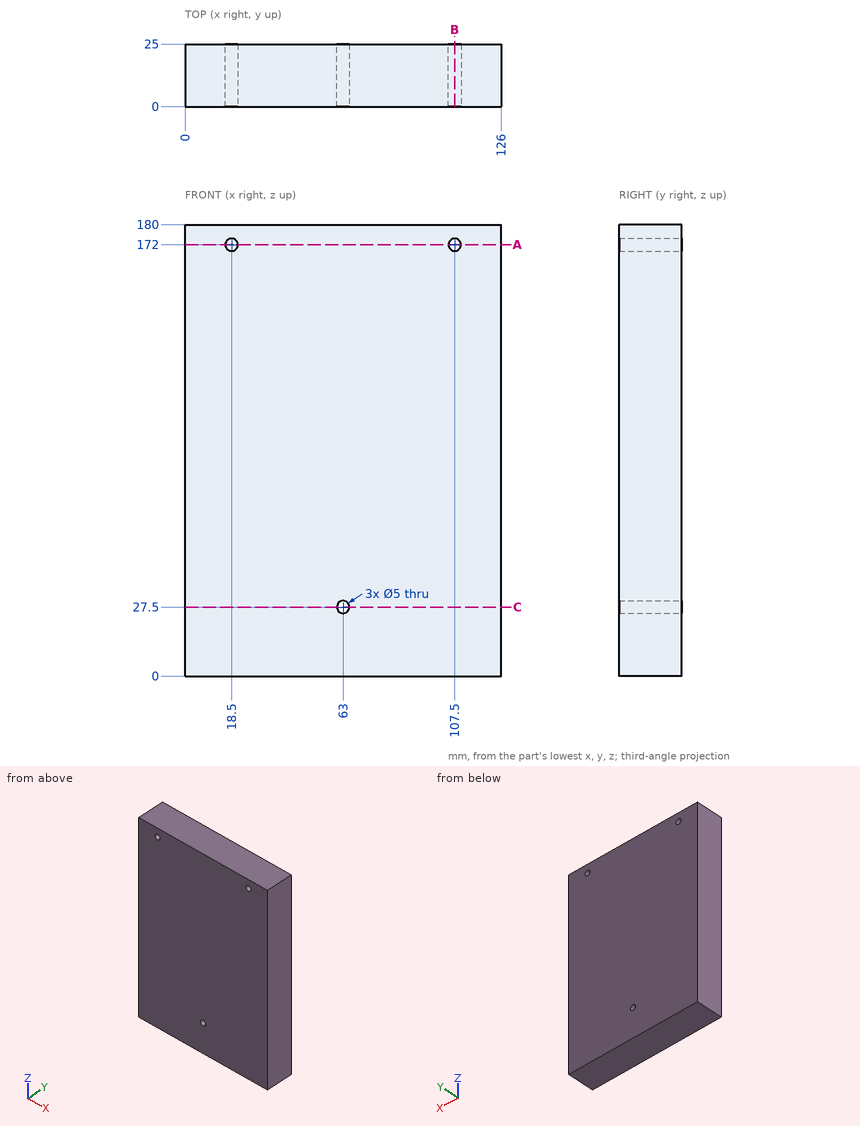
Part print with two shaded views. Sizes in mm from the minimum x, y, z corner. Give positions to 0.01 mm unless a question says otherwise; leave off trailing zeros. Loops run counter-clockwise (first coordinate to the right, second up) from the corner with the lowest first, then second, coordinate; pieces in that order, holes last. Notation, with made-up numbers: (-29.75, 69.5) -> (-9.75, 69.5) arc R33 ccw to (-9.75, 102.5) -> close; hole circle Ø9 at (-28.75, 2). An arc over 180 degrees is marked (long way). One line per question, with ' | ' between items.
Q1. Cut at C-C, the plane z = 27.5. Write the cut outline in (x, y).
Filled sheet:
outline: (0, 0) -> (60.5, 0) -> (60.5, 25) -> (0, 25) -> close; (65.5, 0) -> (126, 0) -> (126, 25) -> (65.5, 25) -> close
Q2. Cut at B-B, the plane x = 107.5. Write the cut outline in (y, z).
Filled sheet:
outline: (0, 0) -> (25, 0) -> (25, 169.5) -> (0, 169.5) -> close; (0, 174.5) -> (25, 174.5) -> (25, 180) -> (0, 180) -> close
Q3. Cut at A-A, the plane z = 172. Write the cut outline in (x, y).
Filled sheet:
outline: (0, 0) -> (16, 0) -> (16, 25) -> (0, 25) -> close; (21, 0) -> (105, 0) -> (105, 25) -> (21, 25) -> close; (110, 0) -> (126, 0) -> (126, 25) -> (110, 25) -> close
Q4. Drill centre lines: line 1 along X through (y, z) = (15, 172); line 2 along Z through (x, y) = (107.5, 12.25); line 3 along Z through (x, y) = (63, 14.25). Where is each one in solid material? Low to high. Write a range as [from, to].
Filled sheet:
line 1: x = [0, 16], [21, 105], [110, 126] | line 2: z = [0, 169.5], [174.5, 180] | line 3: z = [0, 25], [30, 180]
